```python
from build123d import *

# Parameters (mm, degrees)
SKETCH1_R           = 71.12
BOSS_EXTRUDE1_DEPTH = 7.62
FILLET1_R           = 0.9906
SKETCH3_R           = 6.35
BOSS_EXTRUDE2_DEPTH = 7.62
SKETCH5_R           = 6.35
BOSS_EXTRUDE3_DEPTH = 38.1


with BuildPart() as part:
    # Sketch1 → Boss-Extrude1 (new body)
    with BuildSketch(Plane(origin=(0, 0, 0), x_dir=(1, 0, 0), z_dir=(0, 1, 0))):
        with Locations(Location((0, 0, 0), (0, 0, 270))):
            Circle(SKETCH1_R)
    extrude(amount=BOSS_EXTRUDE1_DEPTH)

    # Fillet1
    fillet1_edges = [part.edges().sort_by_distance(p)[0] for p in [
        (0, 0, -71.12),
        (0, 7.62, -71.12),
    ]]
    fillet(fillet1_edges, radius=FILLET1_R)

    # Sketch3 → Boss-Extrude2 (add)
    with BuildSketch(Plane.XY.offset(45.72)):
        with BuildLine():
            Line((0, 0), (43.18, 0))
            Line((43.18, 0), (-61.579637217, -167.864725032))
            ThreePointArc((-61.579637217, -167.864725032), (-100.613254195, -177.896447691), (-112.513352174, -139.391300217))
            Line((-112.513352174, -139.391300217), (-43.18, 0))
            Line((-43.18, 0), (0, 0))
        make_face()
        with Locations((-86.36, -152.4)):
            Circle(SKETCH3_R, mode=Mode.SUBTRACT)
    boss_extrude2 = extrude(amount=BOSS_EXTRUDE2_DEPTH)

    # Mirror1: Boss-Extrude2 across plane
    add(boss_extrude2.mirror(Plane.XY))

    # Sketch5 → Boss-Extrude3 (add)
    with BuildSketch(Plane(origin=(0, 7.62, 0), x_dir=(1, 0, 0), z_dir=(0, 1, 0))):
        with Locations(Location((0, 0, 0), (0, 0, 90))):
            Circle(SKETCH5_R)
    extrude(amount=BOSS_EXTRUDE3_DEPTH)


solid = part.part
```
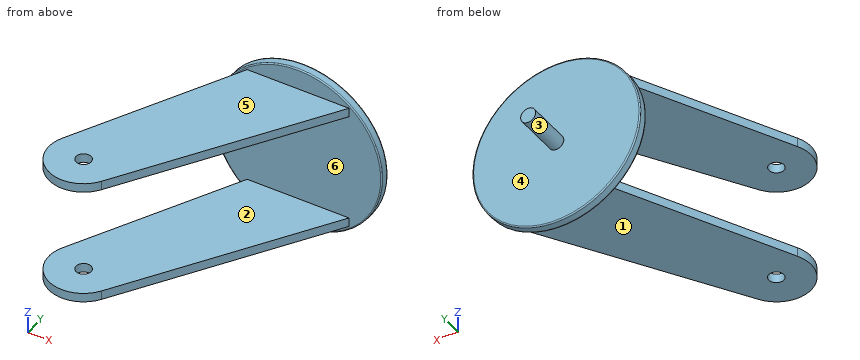
The model under review builds one solid part; all positions refer to its coordinate system, in mm. Face numbers are marked on the shaded views. A direction names the side the tool comes from. Round coordinates to 2 decimals unless told otherwise and drop trailing zeros. Loops run counter-clockwise (first coordinate to the right, second up) from the corner with the lowest first, then second, coordinate; pieces in that order, holes last. Notation, with made-up numbers: (58.25, 76.25) - (90.25, 76.25) arc R28 cw to (90.25, 100.25) - close; hole circle Ø10 at (51, 8). An arc over 180 degrees is marked (long way). Use a Markdown table: item, result. Add a question column.
Q1. Add section A-A (y = -51.5). State the section outline as (x, z) points, plus the area to 3 significant figures.
Q2. The part is to be moulded in two halves that separate along Z. For the marked faces 4, 5 and 6, say which applies: pulls with the +Z half, pulls with the -Z half, needs draft (parallel to the pull), parting line crosses it, or undercut.
Q3. Add section D-D (y = -152.4). State the section outline as (x, z) points, plus the area to 3 significant figures.
Q4. Insertion check: pin 1 Ø2 at (y, z) = (-19.5, 43) entering from +X; pin 2 Ø12 at (x, z) = (2, -13.5) entering from -Y; pin 3 Ø14.5 at (x, y) = (-86.36, -152.4) entering from -Z; pin 4 Ø8 at (x, z) = (-26, -1.5) entering from +Y. Each pin has a flat end and moves straight along its axis. Give the tip position at first contact, or say it passes through.
Q5. Add section C-C (x = -86.36). State the section outline as (y, z) points, plus the area to 3 significant figures.
Q6. Machinability: for the marked faces 1, 2 and 3, which of the approach directions +Z, -Z, +X, -X, +Y, -Y give a long, thin tool a straight path to every point of the face, cutting with its end or side? Answer none if there is none.
Q7. For probe 1 along Z at (x, y) = (-88.5, -163.5); probe 2 along Y at (x, z) = (47, -5.5); probe 3 along Y at (x, z) = (-86, 48), list the stretches that pass through material, from the lowest coordinate up.
Q8. Add section B-B (z = 0). State the section outline as (x, y) points, plus the area to 3 significant figures.
Worked answers:
| question | item | result |
|---|---|---|
| 1 | outline | (-68.8, -53.34) - (11.04, -53.34) - (11.04, -45.72) - (-68.8, -45.72) - close; (-68.8, 45.72) - (11.04, 45.72) - (11.04, 53.34) - (-68.8, 53.34) - close |
| 1 | area | 1,220 mm² |
| 2 | face 4 | needs draft |
| 2 | face 5 | pulls with the +Z half |
| 2 | face 6 | undercut |
| 3 | outline | (-115.57, -53.34) - (-92.71, -53.34) - (-92.71, -45.72) - (-115.57, -45.72) - close; (-115.57, 45.72) - (-92.71, 45.72) - (-92.71, 53.34) - (-115.57, 53.34) - close; (-80.01, -53.34) - (-51.93, -53.34) - (-51.93, -45.72) - (-80.01, -45.72) - close; (-80.01, 45.72) - (-51.93, 45.72) - (-51.93, 53.34) - (-80.01, 53.34) - close |
| 3 | area | 776 mm² |
| 4 | pin 1 | through |
| 4 | pin 2 | y = 0 |
| 4 | pin 3 | z = -53.34 |
| 4 | pin 4 | y = 7.62 |
| 5 | outline | (-181.61, -53.34) - (-158.75, -53.34) - (-158.75, -45.72) - (-181.61, -45.72) - close; (-181.61, 45.72) - (-158.75, 45.72) - (-158.75, 53.34) - (-181.61, 53.34) - close; (-146.05, -53.34) - (-86.81, -53.34) - (-86.81, -45.72) - (-146.05, -45.72) - close; (-146.05, 45.72) - (-86.81, 45.72) - (-86.81, 53.34) - (-146.05, 53.34) - close |
| 5 | area | 1,250 mm² |
| 6 | face 1 | -Z, +X, -X, -Y |
| 6 | face 2 | +X, -X, -Y |
| 6 | face 3 | +Y |
| 7 | probe 1 | -53.34 to -45.72, 45.72 to 53.34 |
| 7 | probe 2 | 0 to 7.62 |
| 7 | probe 3 | -181.61 to -158.74, -146.06 to -86.09 |
| 8 | outline | (-71.12, 0.99) arc R0.99 ccw to (-70.13, 0) - (70.13, 0) arc R0.99 ccw to (71.12, 0.99) - (71.12, 6.63) arc R0.99 ccw to (70.13, 7.62) - (6.35, 7.62) - (6.35, 45.72) - (-6.35, 45.72) - (-6.35, 7.62) - (-70.13, 7.62) arc R0.99 ccw to (-71.12, 6.63) - close |
| 8 | area | 1,570 mm² |
